The model under review builds one solid part; all positions refer to its coordinate system, in mm. Face numbers are marked on the shaded views. Coordinates: 2 decimals unless noted, no trailing zeros. Write each loop counter-clockwise with the first axis right and the second up, starting at its lowest first coordinate (ties: lowest second). Pieces come first, ordered by that corner, then holes. Notation, with made-up numbers: (-11, 22.5) - (43, 22.5) arc R21 cw to (43, 60.5) - close; hole circle Ø4 at (61.25, 39.25). An arc over 180 degrees is marked (long way). Answer as CSV lines item,"result". Start each with the question number.
```python
from build123d import *

# Parameters (mm, degrees)
SKETCH1_R           = 6.6675
BOSS_EXTRUDE1_DEPTH = 20.32
SKETCH4_R           = 3.048
BOSS_EXTRUDE2_DEPTH = 83.82
SKETCH5_R           = 4.191
BOSS_EXTRUDE3_DEPTH = 12.7
FILLET1_R           = 0.508


with BuildPart() as part:
    # Sketch1 → Boss-Extrude1 (new body)
    with BuildSketch(Plane(origin=(0, 0, 0), x_dir=(1, 0, 0), z_dir=(0, 1, 0))):
        with Locations(Location((0, 0, 0), (0, 0, 270))):
            Circle(SKETCH1_R)
    extrude(amount=BOSS_EXTRUDE1_DEPTH)

    # Loft1: read off the stored shape, not the designer's step
    # Loft1: loft between two sections, ruled curve by curve
    loft1_from = [
        Edge.make_bspline([(0.590355185, 64.77, -2.990281719), (6.570918622, 64.77, -1.809571349), (5.390208252, 64.77, 4.170992088), (-0.590355185, 64.77, 2.990281719), (-6.570918622, 64.77, 1.809571349), (-5.390208252, 64.77, -4.170992088), (0.590355185, 64.77, -2.990281719)], [0, 0, 0, 0, 0.5, 0.5, 0.5, 1, 1, 1, 1], 3, [1, 0.333333333, 0.333333333, 1, 0.333333333, 0.333333333, 1]),
    ]
    loft1_to = [
        Edge.make_bspline([(3.019513857, 20.32, -5.944585126), (14.908684109, 20.32, 0.094442589), (8.869656394, 20.32, 11.98361284), (-3.019513857, 20.32, 5.944585126), (-14.908684109, 20.32, -0.094442589), (-8.869656394, 20.32, -11.98361284), (3.019513857, 20.32, -5.944585126)], [0, 0, 0, 0, 0.5, 0.5, 0.5, 1, 1, 1, 1], 3, [1, 0.333333333, 0.333333333, 1, 0.333333333, 0.333333333, 1]),
    ]
    loft1 = Solid(Shell([*[Face.make_surface_from_curves(loft1_from[k], loft1_to[k]) for k in range(1)], Face(Wire(loft1_from)), Face(Wire(loft1_to))]))
    add(loft1)

    # Sketch4 → Boss-Extrude2 (add)
    with BuildSketch(Plane(origin=(0, 64.77, 0), x_dir=(1, 0, 0), z_dir=(0, 1, 0))):
        with Locations(Location((0, 0, 0), (0, 0, 78.832021496))):
            Circle(SKETCH4_R)
    extrude(amount=BOSS_EXTRUDE2_DEPTH)

    # Sketch5 → Boss-Extrude3 (add)
    with BuildSketch(Plane(origin=(0, 148.59, 0), x_dir=(1, 0, 0), z_dir=(0, 1, 0))):
        with Locations(Location((0, 0, 0), (0, 0, 270))):
            Circle(SKETCH5_R)
    extrude(amount=BOSS_EXTRUDE3_DEPTH)

    # Fillet1
    fillet1_edges = [part.edges().sort_by_distance(p)[0] for p in [
        (0, 148.59, -4.191),
        (0, 161.29, -4.191),
        (0, 0, -6.6675),
        (6.48425314, 20.32, 1.552423094),
    ]]
    fillet(fillet1_edges, radius=FILLET1_R)


solid = part.part
```
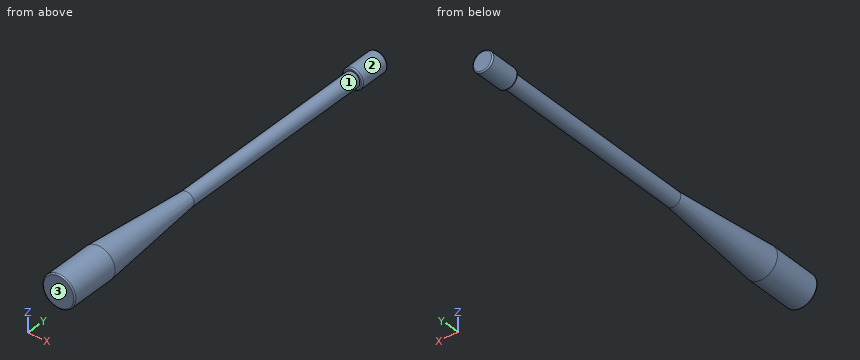
(1) The part is to be moulded in two halves that separate along Y. For the marked faces 1, 2 and 3, say which applies: released by +Y, released by -Y, zero draft, split by the parting line, or undercut.
(2) Add section A-A on y = 13. Give the boundary of the cut face in (x, z) (1 decimal).
(3) Wall thickness on line 1 (Z direction, x = 0.25, y = 154.5); line 2 (Z direction, x = -0.25, y = 148); line 3 (X direction, y = 97.5, z = -2.5): over which ranges is each line inside the solid? List them lowest first.
(4) For pin 1 (4 mm diameter, centred on x = -2, z = -2, fed in from -Y); pin 2 (5 mm diameter, centred on y = 119.5, z = 3, fed in from -X); pin 3 (6 mm diameter, centred on y = 25.5, z = -5, fed in from +X); pin 4 (1.5 mm diameter, centred on y = 134.5, z = -2.5, fed in from +X), all flat-tipped, find the tip position at first contact; note any pin that passes through.
Reported:
1,face 1,"undercut"
1,face 2,"zero draft"
1,face 3,"released by -Y"
2,outline,"circle Ø13.3 at (0, 0)"
3,line 1,"-4.18 to 4.18"
3,line 2,"-3.04 to 3.04"
3,line 3,"-1.74 to 1.74"
4,pin 1,"y = 0"
4,pin 2,"x = -3.01"
4,pin 3,"x = 5.94"
4,pin 4,"x = 2.5"
